from build123d import *

# Parameters (mm, degrees)
SKETCH1_R           = 18.5
BOSS_EXTRUDE1_DEPTH = 20
SKETCH2_R           = 20
BOSS_EXTRUDE2_DEPTH = 2
SKETCH3_R           = 20
BOSS_EXTRUDE3_DEPTH = 2
CUT_EXTRUDE1_DEPTH  = 21


with BuildPart() as part:
    # Sketch1 → Boss-Extrude1 (new body)
    with BuildSketch(Plane.XY):
        Circle(SKETCH1_R)
    extrude(amount=BOSS_EXTRUDE1_DEPTH)

    # Sketch2 → Boss-Extrude2 (add)
    with BuildSketch(Plane.XY.offset(20)):
        Circle(SKETCH2_R)
    extrude(amount=-BOSS_EXTRUDE2_DEPTH)

    # Sketch3 → Boss-Extrude3 (add)
    with BuildSketch(Plane(origin=(0, 0, 0), x_dir=(-1, 0, 0), z_dir=(0, 0, -1))):
        Circle(SKETCH3_R)
    extrude(amount=-BOSS_EXTRUDE3_DEPTH)

    # Sketch4 → Cut-Extrude1 (cut, through all)
    with BuildSketch(Plane.XY.offset(20)):
        Polygon((5.772232155, 4.521578185), (-1.029685496, 7.259688775), (-6.801917651, 2.73811059), (-5.772232155, -4.521578185), (1.029685496, -7.259688775), (6.801917651, -2.73811059), align=None)
    extrude(amount=-CUT_EXTRUDE1_DEPTH, mode=Mode.SUBTRACT)


solid = part.part
Model file for the job. Use its own axes, mm. A direction names the side the tool comes from. Coordinates: 2 decimals unless noted, no trailing zeros. Write each loop counter-clockwise with the first axis right and the second up, starting at its lowest first coordinate (ties: lowest second). Pieces come first, ordered by that corner, then holes. Notation, with made-up numbers: (-24.75, 35) -> (19.25, 35) arc R22 cw to (19.25, 56) -> close; hole circle Ø11 at (-23, 36). An arc over 180 degrees is marked (long way). One line per item, written item: value. Start each with the question number.
1) Slice it at A-A on z = 10.25. Write the cut outline in (x, y).
2) Which spindle directions (+Z, -Z, +X, -X, +Y, -Y) get a long thin tool onto all of the face, cutting with end or side? Do faces 4 (the face through (6.3, 0.8, 10.1)), 5 (the face through (-6, -18, 2)), 6 (the face through (0, -9, 0)). Say none if no direction does.
3) Slice it at D-D on x = -13. Write the cut outline in (y, z).
4) Probe probe 1 along X at (y, z) = (-5, 4.5); probe 2 along Y at (x, z) = (3, 17.5); probe 3 along Y at (x, z) = (4.5, 13.75). List the from-to ranges inside material, lowest first.
5) Pull direction Y, two halves, no side cores. Call faces 1 (the face through (-6.3, -0.8, 10.1)), 2 (the face through (-5, 5, 20)), 3 (the face through (-4.01, -18.06, 9.89)): +Y half, -Y half, draft (parallel to the pull), parting line (faces both ways), or undercut.
6) Slice it at B-B on y = 4. Write the cut outline in (x, z), then the cut area to 3 significant figures.
7) Slice it at C-C on x = -4.5. Write the cut outline in (y, z).
8) Flat gauge pins, fed straight in: pin 1 Ø4 at (x, z) = (5, 9) entering from -Y; pin 2 Ø8 at (x, z) = (-7.5, 11) entering from -Y; pin 3 Ø1 at (y, z) = (6, 8.5) entering from -X. Where does each tip first touch, or does it go through?
Answers follow:
1. outline: circle Ø37 at (0, 0); hole (-6.8, 2.74) -> (-5.77, -4.52) -> (1.03, -7.26) -> (6.8, -2.74) -> (5.77, 4.52) -> (-1.03, 7.26) -> close
2. face 4: +Z, -Z
2. face 5: none
2. face 6: -Z, +X, -X, +Y, -Y
3. outline: (-15.2, 0) -> (15.2, 0) -> (15.2, 2) -> (13.16, 2) -> (13.16, 18) -> (15.2, 18) -> (15.2, 20) -> (-15.2, 20) -> (-15.2, 18) -> (-13.16, 18) -> (-13.16, 2) -> (-15.2, 2) -> close
4. probe 1: -17.81 to -4.58, 3.91 to 17.81
4. probe 2: -18.26 to -5.72, 5.64 to 18.26
4. probe 3: -17.94 to -4.54, 5.03 to 17.94
5. face 1: undercut
5. face 2: draft
5. face 3: parting line
6. outline: (-19.6, 0) -> (-5.19, 0) -> (-5.19, 20) -> (-19.6, 20) -> (-19.6, 18) -> (-18.06, 18) -> (-18.06, 2) -> (-19.6, 2) -> close; (5.85, 0) -> (19.6, 0) -> (19.6, 2) -> (18.06, 2) -> (18.06, 18) -> (19.6, 18) -> (19.6, 20) -> (5.85, 20) -> close
6. area: 514 mm2
7. outline: (-19.49, 0) -> (-5.03, 0) -> (-5.03, 20) -> (-19.49, 20) -> (-19.49, 18) -> (-17.94, 18) -> (-17.94, 2) -> (-19.49, 2) -> close; (4.54, 0) -> (19.49, 0) -> (19.49, 2) -> (17.94, 2) -> (17.94, 18) -> (19.49, 18) -> (19.49, 20) -> (4.54, 20) -> close
8. pin 1: y = -18.26
8. pin 2: y = -18.17
8. pin 3: x = -17.66
